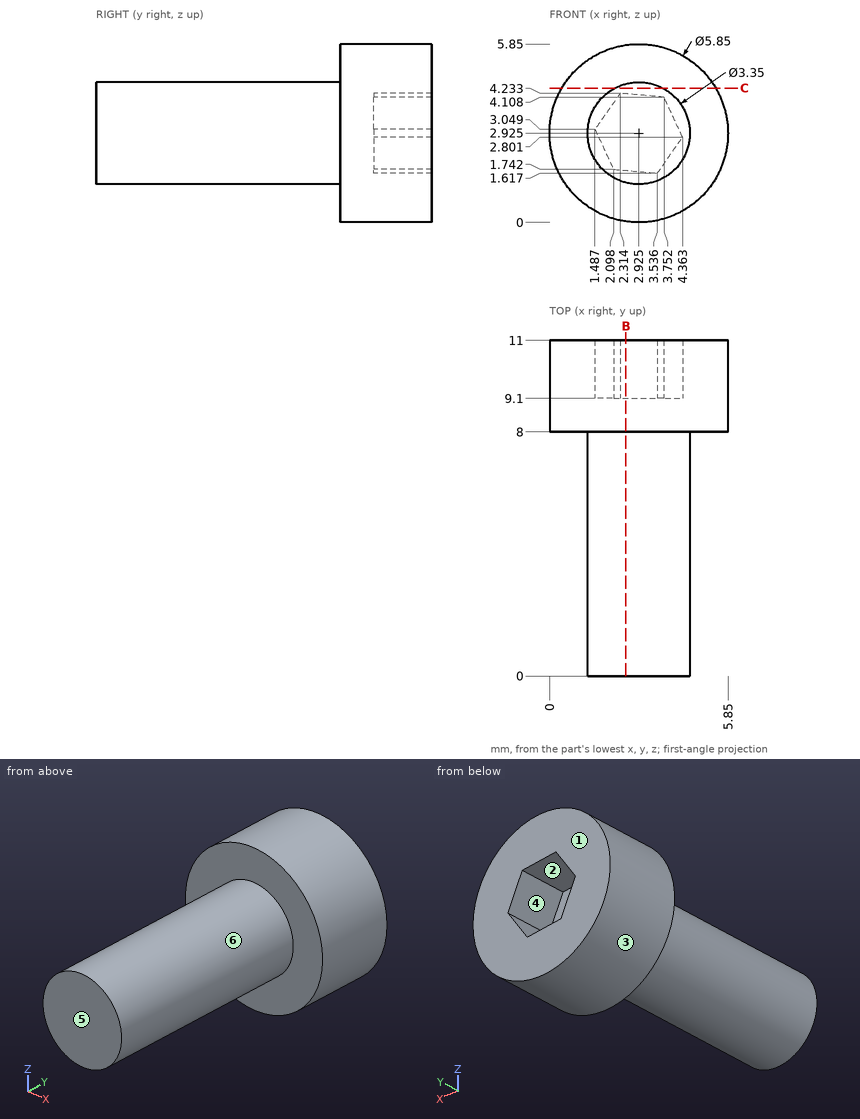
Could you check a few things on this drawing? It's one solid part, dimensions in mm from its lowest x, y, z. A direction names the side the tool comes from. Coordinates: 2 decimals unless noted, no trailing zeros. Order: outer loops, then holes, each group sorted by start corner. A loop starts at its lowest first (then second) coordinate and runs counter-clockwise, first axis right, second up. Notation, with made-up numbers: M 68.5,7 L 81.5,7 A18 cw 81.5,26 Z; hole C 70.5,36 d8. An arc over 180 degrees is marked long. Use a Markdown table: item, result. Add a question column.
Q1. We'd pull the mould along Z, two halves only. Please class the marked faces 1, 2, 3 and 4: pulls with the +Z half, pulls with the -Z half, needs draft (parallel to the pull), parting line crosses it, or undercut.
Q2. I'm going to push flat-ended pins straight in: pin 1 (2 mm diameter, centred on y = 9.5, z = 0.5, fed in from -X); pin 2 (3 mm diameter, centred on x = 3.5, z = 1, fed in from -Y); pin 3 (1 mm diameter, centred on y = 1, z = 2.5, fed in from -X); pin 4 (2 mm diameter, centred on x = 3, y = 6.5, fed in from +Z). Where does each tip first touch, or does it pass through?
Q3. Which directions (+Z, -Z, +X, -X, +Y, -Y) give clear straight access to the entire face, cutting with the end or side of a thin tool? Please do the marked faces 5 and 6.
Q4. If I drill on L1, parallel to Y at x = 2.05, z = 5.2; L2, parallel to Z at x = 3.3, y = 9.5 (1 decimal); L3, parallel to X at y = 8.75, z = 1.8 (1 decimal), over which ranges is the centre line in solid material (lowest first)?
Q5. I want a section at C-C on z = 4.4. List the corners of the cut face in (x, y) for me.
Q6. I want a section at B-B on x = 2.5. List the corners of the cut face in (y, z) for me (1 decimal), then the cut area to 3 significant figures.
Checked values:
| question | item | result |
|---|---|---|
| 1 | face 1 | needs draft |
| 1 | face 2 | undercut |
| 1 | face 3 | parting line crosses it |
| 1 | face 4 | undercut |
| 2 | pin 1 | x = 0.37 |
| 2 | pin 2 | y = 0 |
| 2 | pin 3 | x = 1.25 |
| 2 | pin 4 | z = 4.6 |
| 3 | face 5 | +Z, -Z, +X, -X, -Y |
| 3 | face 6 | -Y |
| 4 | L1 | 8 to 11 |
| 4 | L2 | 0 to 1.6, 4.1 to 5.8 |
| 4 | L3 | 0.2 to 5.6 |
| 5 | outline | M 0.4,8 L 2.13,8 L 2.13,0 L 3.72,0 L 3.72,8 L 5.45,8 L 5.45,11 L 0.4,11 Z |
| 6 | outline | M 0,1.3 L 8,1.3 L 8,0 L 11,0 L 11,1.7 L 9.1,1.7 L 9.1,4.2 L 11,4.2 L 11,5.8 L 8,5.8 L 8,4.5 L 0,4.5 Z |
| 6 | area | 38.5 mm² |
